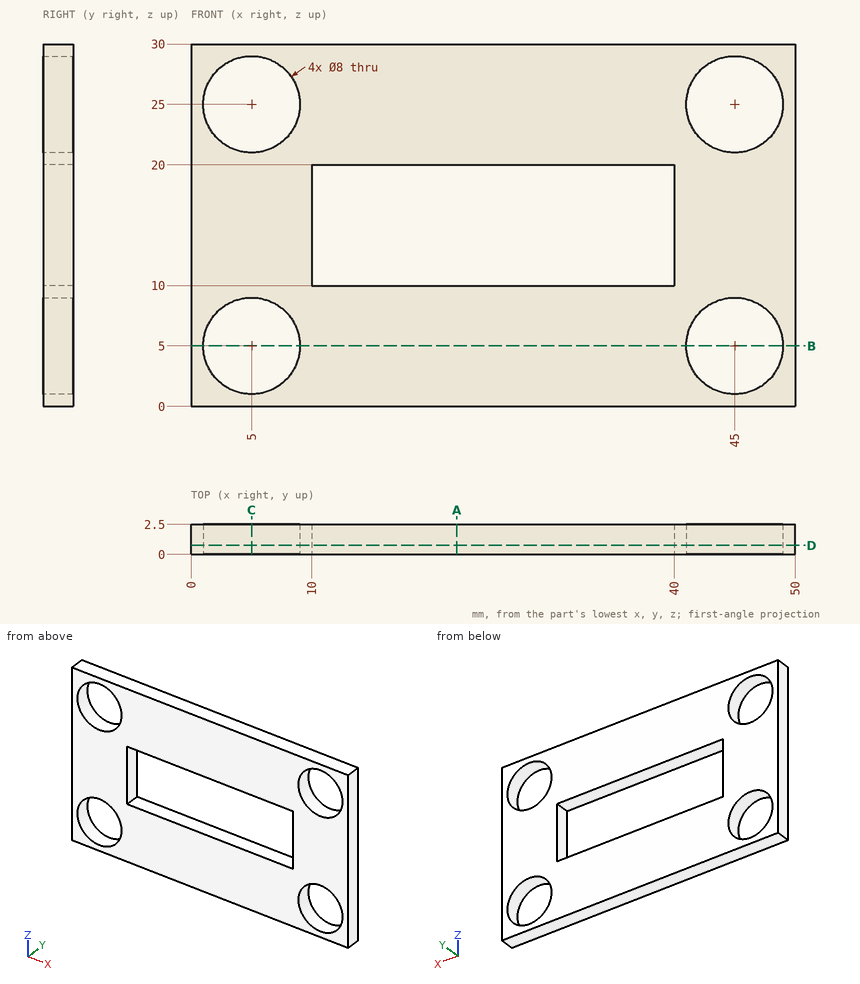
Design review of the part shown in the three views and the two pictorial views. Dimensions are in mm from the part's minimum x, y and z. Round coordinates to 2 decimals unless told otherwise and drop trailing zeros. Order: outer loops, then holes, each group sorted by start corner. A loop starts at its lowest first (then second) coordinate and runs counter-clockwise, first axis right, second up. Notation, with made-up numbers: M -12,-17.5 L 17,-17.5 A26 cw 17,21.5 Z; hole C 80.25,68 d11. An arc over 180 degrees is marked long. Put each result on its own line as item: value.
Q1. Consider section D-D (y = 0.75). State the section outline as (x, z) points, and give its area (3 significant figures).
Reported:
outline: M 0,0 L 50,0 L 50,30 L 0,30 Z; hole C 5,5 d8; hole C 5,25 d8; hole M 10,10 L 40,10 L 40,20 L 10,20 Z; hole C 45,5 d8; hole C 45,25 d8
area: 999 mm²
Q2. Consider section C-C (x = 5). State the section outline as (y, z) points, and give its area (3 significant figures).
Reported:
outline: M 0,0 L 2.5,0 L 2.5,1 L 0,1 Z; M 0,9 L 2.5,9 L 2.5,21 L 0,21 Z; M 0,29 L 2.5,29 L 2.5,30 L 0,30 Z
area: 35.0 mm²
Q3. Insertion check: pin 1 Ø9 at (x, z) = (45, 5) entering from +Y; pin 2 Ø5 at (x, z) = (14.5, 13) entering from +Y. Each pin has a flat end and moves straight along its axis. Give the tip position at first contact, or say it passes through.
Reported:
pin 1: y = 2.5
pin 2: through
Q4. Consider section A-A (x = 22). State the section outline as (y, z) points.
Reported:
outline: M 0,0 L 2.5,0 L 2.5,10 L 0,10 Z; M 0,20 L 2.5,20 L 2.5,30 L 0,30 Z
Q5. Consider section B-B (z = 5). State the section outline as (x, y) points, and give its area (3 significant figures).
Reported:
outline: M 0,0 L 1,0 L 1,2.5 L 0,2.5 Z; M 9,0 L 41,0 L 41,2.5 L 9,2.5 Z; M 49,0 L 50,0 L 50,2.5 L 49,2.5 Z
area: 85.0 mm²
Q6. To check wall thickness, follow line 1 (X direction, y = 1.25, z = 25); line 2 (Z direction, x = 15, y = 1.05); line 3 (X direction, y = 1.1, z = 6.25). State the ranges of each line that lie inside material, in increasing order.
Reported:
line 1: 0 to 1, 9 to 41, 49 to 50
line 2: 0 to 10, 20 to 30
line 3: 0 to 1.2, 8.8 to 41.2, 48.8 to 50
